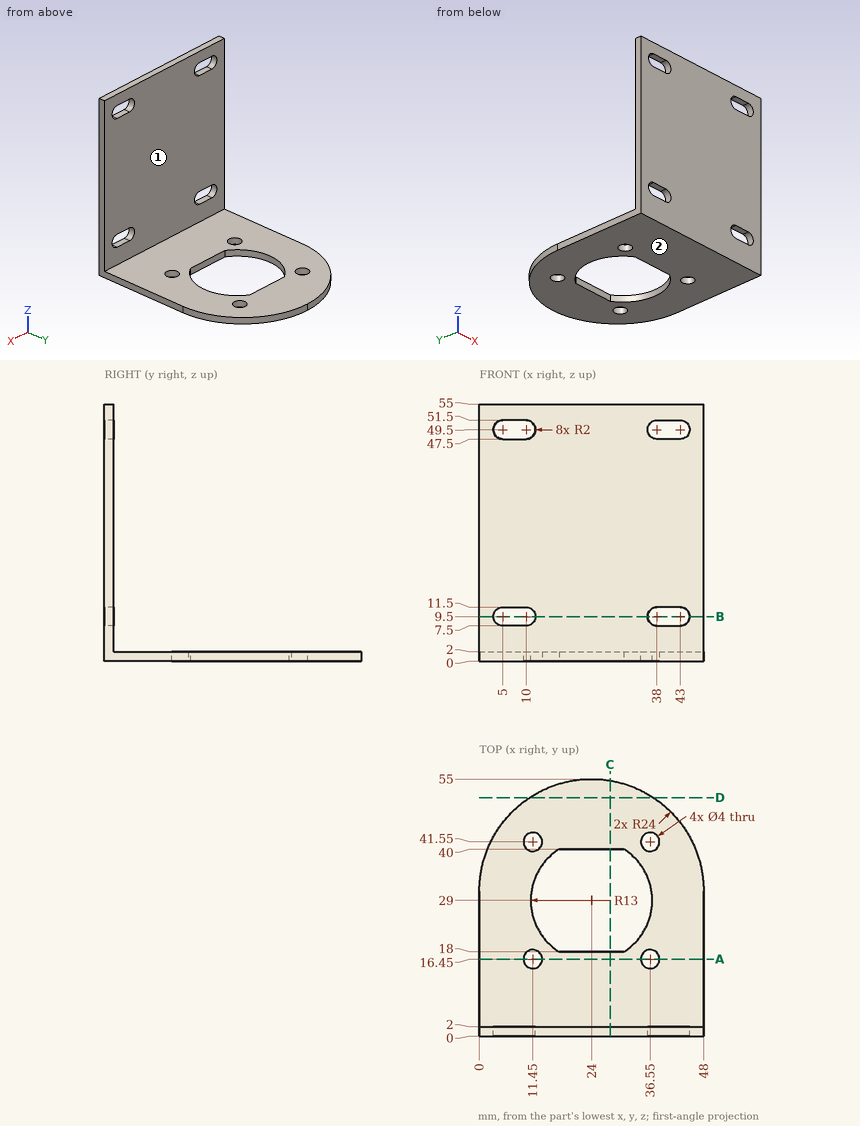
Geometry check sheet. Reference: drawing and pictorial views, mm from the part's lowest x, y, z. A direction names the side the tool comes from. Round coordinates to 2 decimals unless told otherwise and drop trailing zeros. Loops run counter-clockwise (first coordinate to the right, second up) from the corner with the lowest first, then second, coordinate; pieces in that order, holes last. Notation, with made-up numbers: M 34,70 L 52,70 A34 cw 52,101 Z; hole C 76,63.25 d3. An arc over 180 degrees is marked long. Return JSON: item names as keys, results as strings. Group by question number.
(1) Section check B-B, the plane z = 9.5. Enter the section's corners in (x, y).
(2) Section check A-A, the plane y = 16.45. Enter the section's corners in (x, z).
(3) Section check D-D, the plane y = 51. Enter the section's corners in (x, z).
(4) Scan line: line 1 along Y through (x, z) = (5.5, 30). Record every from-to range of solid material in increasing order. Write a range as [from, to].
(5) Set-up check for the marked faces 1 and 2: record each of +Z, -Z, +X, -X, +Y, -Y from which the full face is reachable in a straight line by a thin tool's end or side.
(6) Section check C-C, the plane x = 28. Enter the section's corners in (y, z), and give its area (3 significant figures).
(7) Go/stop test with flat-tipped pins: pin 1 (10 mm diameter, centred on x = 12.5, y = 7.5, fed in from -Z); pin 2 (1.6 mm diameter, centred on x = 27, z = 1, fed in from +Y); pin 3 (6 mm diameter, centred on x = 17, y = 8.5, fed in from +Z); pin 4 (24 mm diameter, centred on x = 27.5, z = 17, fed in from +Y). Record where each tip stops, or that it passes through.
Data:
{
 "1": {"outline": "M 0,0 L 3,0 L 3,2 L 0,2 Z; M 12,0 L 36,0 L 36,2 L 12,2 Z; M 45,0 L 48,0 L 48,2 L 45,2 Z"},
 "2": {"outline": "M 0,0 L 9.45,0 L 9.45,2 L 0,2 Z; M 13.45,0 L 34.55,0 L 34.55,2 L 13.45,2 Z; M 38.55,0 L 48,0 L 48,2 L 38.55,2 Z"},
 "3": {"outline": "M 10.73,0 L 37.27,0 L 37.27,2 L 10.73,2 Z"},
 "4": {"line 1": "[0, 2]"},
 "5": {"face 1": "+Z, +X, -X, +Y", "face 2": "-Z, +X, -X, +Y, -Y"},
 "6": {"outline": "M 0,0 L 18,0 L 18,2 L 2,2 L 2,55 L 0,55 Z; M 40,0 L 54.66,0 L 54.66,2 L 40,2 Z", "area": "171 mm²"},
 "7": {"pin 1": "z = 0", "pin 2": "y = 54.9", "pin 3": "z = 2", "pin 4": "y = 2"}
}
